Geometry: final body of the model. Coordinates: model frame, mm. A direction names the side the tool comes from. Give positions to 0.01 mm unless a question says otherwise; leave off trailing zeros. Write each loop counter-clockwise with the first axis right and the second up, starting at its lowest first coordinate (ties: lowest second). Pieces come first, ordered by that corner, then holes. Notation, with made-up numbers: (-3, -12.75) -> (43, -12.75) arc R23 cw to (43, 25.25) -> close; hole circle Ø6 at (35, 50.25). An arc over 180 degrees is marked (long way). Use CSV: the item, a comma, the result in double quotes. Start each with the question number.
1) Section D-D (z = 3.5). Output: boundary loops of the cut face in (x, y), plus the area to 3 significant figures.
2) Section A-A (z = 6). Output: boundary loops of the cut face in (x, y), plus the area to 3 significant figures.
3) Section C-C (x = 6.5). Output: boundary loops of the cut face in (y, z), plus the area to 3 significant figures.
4) Contact query for flat-ended pins moving along their axis: P1, Ø1.5, axis at x = -9, z = 10.5, coming from the -Y side; P2, Ø4, axis at x = 10, y = 6, coming from the +Z side; P3, Ø4, axis at x = -7.53, y = 0, coming from the -Z side; P4, Ø2.5, axis at y = -8, z = -3.5, coming from the +X side. Output: stop coordinate, or through.
5) Material intervals for line 1 (X direction, y = 10, z = 6.5); line 2 (X direction, y = 7.25, z = 6.75); line 3 (X direction, y = -0.75, z = 1), sorted ascending. Write a range as [from, to].
6) Draft query along X for faces 4 (the face through (9.432, -3, 1)), 5 (the face through (0.332, -7.4, -4.5)), 6 (the face through (-3.81, -10, -1)). Return one class per face: pulls with the +X half, pulls with the -X half, needs draft (parallel to the pull), parting line crosses it, or undercut.
7) Section B-B (y = 0). Output: boundary loops of the cut face in (x, z).
8) Set-up query: faces 1 (the face through (11.34, 8.13, 2.98)), 2 (the face through (3, -8.46, -1)), 3 (the face through (0, -9, -2.54)). Return all of +Z, -Z, +X, -X, +Y, -Y with unobstructed straight access to the full face (end or side cutting, diameter ignored); none if empty.
```python
from build123d import *

# Parameters (mm, degrees)
IZIM1_R                     = 1.900647948
IZIM1_R_2                   = 1.75
Y_KSEKLIK_EKSTR_ZYON1_DEPTH = 1.7
IZIM2_R                     = 2
Y_KSEKLIK_EKSTR_ZYON2_DEPTH = 2.6
IZIM3_W                     = 4.100055298
IZIM3_H                     = 6.937365011
Y_KSEKLIK_EKSTR_ZYON3_DEPTH = 8.5
IZIM4_W                     = 5.8
IZIM4_H                     = 6.937365011
Y_KSEKLIK_EKSTR_ZYON4_DEPTH = 0.6
Y_KSEKLIK_EKSTR_ZYON6_DEPTH = 2.54
IZIM6_W                     = 18.863930886
IZIM6_H                     = 1.7
Y_KSEKLIK_EKSTR_ZYON7_DEPTH = 0.01
KES_EKSTR_ZYON1_DEPTH       = 5.9
KES_EKSTR_ZYON1_DEPTH_BACK  = 0.1
IZIM7_W                     = 6.75
IZIM7_H                     = 0.75
IZIM8_W                     = 0.664910116
IZIM8_H                     = 0.664910116
IZIM11_W                    = 0.65
IZIM11_H                    = 0.6
Y_KSEKLIK_EKSTR_ZYON8_DEPTH = 1
Y_KSEKLIK_EKSTR_ZYON9_DEPTH = 1.5


with BuildPart() as part:
    # Çizim1 → Yükseklik-Ekstrüzyon1 (new body)
    with BuildSketch(Plane.XY):
        with BuildLine():
            Line((-9.431965443, -11), (9.431965443, -11))
            Line((9.431965443, -11), (9.431965443, 4.062634989))
            ThreePointArc((9.431965443, 4.062634989), (12.900647948, 7.531317495), (9.431965443, 11))
            Line((9.431965443, 11), (-9.431965443, 11))
            ThreePointArc((-9.431965443, 11), (-12.900647948, 7.531317495), (-9.431965443, 4.062634989))
            Line((-9.431965443, 4.062634989), (-9.431965443, -11))
        make_face()
        with Locations((9.431965443, 7.531317495)):
            Circle(IZIM1_R, mode=Mode.SUBTRACT)
        with Locations(Location((-9.431965443, 7.531317495, 0), (0, 0, 180))):
            Circle(IZIM1_R, mode=Mode.SUBTRACT)
        with Locations((7.531317495, 0)):
            Circle(IZIM1_R_2, mode=Mode.SUBTRACT)
        with Locations(Location((-7.531317495, 0, 0), (0, 0, 180))):
            Circle(IZIM1_R_2, mode=Mode.SUBTRACT)
    extrude(amount=Y_KSEKLIK_EKSTR_ZYON1_DEPTH)

    # Çizim2 → Yükseklik-Ekstrüzyon2 (add)
    with BuildSketch(Plane.XY.offset(1.7)):
        with BuildLine():
            Line((-9.431965443, 11), (9.431965443, 11))
            ThreePointArc((9.431965443, 11), (12.900647948, 7.531317495), (9.431965443, 4.062634989))
            Line((9.431965443, 4.062634989), (-9.431965443, 4.062634989))
            ThreePointArc((-9.431965443, 4.062634989), (-12.900647948, 7.531317495), (-9.431965443, 11))
        make_face()
        with Locations((-9.431965443, 7.531317495)):
            Circle(IZIM2_R, mode=Mode.SUBTRACT)
        with Locations((9.431965443, 7.531317495)):
            Circle(IZIM2_R, mode=Mode.SUBTRACT)
    extrude(amount=Y_KSEKLIK_EKSTR_ZYON2_DEPTH)

    # Çizim3 → Yükseklik-Ekstrüzyon3 (add)
    with BuildSketch(Plane.XY.offset(4.3)):
        with Locations((4.950027649, 7.531317494)):
            Rectangle(IZIM3_W, IZIM3_H)
        with Locations((-4.950027649, 7.531317494)):
            Rectangle(IZIM3_W, IZIM3_H)
    extrude(amount=Y_KSEKLIK_EKSTR_ZYON3_DEPTH)

    # Çizim4 → Yükseklik-Ekstrüzyon4 (add)
    with BuildSketch(Plane.XY.offset(4.3)):
        with Locations((0, 7.531317494)):
            Rectangle(IZIM4_W, IZIM4_H)
    extrude(amount=Y_KSEKLIK_EKSTR_ZYON4_DEPTH)

    # Çizim5 → Yükseklik-Ekstrüzyon6 (add)
    with BuildSketch(Plane(origin=(0, 0, 0), x_dir=(-1, 0, 0), z_dir=(0, 0, -1))):
        Polygon((-1.27, -10.75), (-1.27, -8.71), (-1.52, -8.46), (-3.56, -8.46), (-3.81, -8.71), (-3.81, -10.75), (-3.56, -11), (-1.52, -11), align=None)
        Polygon((1.27, -8.71), (1.02, -8.46), (-1.02, -8.46), (-1.27, -8.71), (-1.27, -10.75), (-1.02, -11), (1.02, -11), (1.27, -10.75), align=None)
        Polygon((1.52, -8.46), (1.27, -8.71), (1.27, -10.75), (1.52, -11), (3.56, -11), (3.81, -10.75), (3.81, -8.71), (3.56, -8.46), align=None)
    extrude(amount=Y_KSEKLIK_EKSTR_ZYON6_DEPTH)

    # Çizim6 → Yükseklik-Ekstrüzyon7 (add)
    with BuildSketch(Plane.XZ.offset(11)):
        with Locations((0, 0.85)):
            Rectangle(IZIM6_W, IZIM6_H)
    extrude(amount=Y_KSEKLIK_EKSTR_ZYON7_DEPTH)

    # Çizim7 → Kes-Ekstrüzyon1 (cut, two sides: drawn at the far end of the back side and taken through both)
    with BuildSketch(Plane.ZY.offset(-2.9).offset(-KES_EKSTR_ZYON1_DEPTH_BACK)):
        with Locations((8.275, 7.531317495)):
            Rectangle(IZIM7_W, IZIM7_H)
    extrude(amount=KES_EKSTR_ZYON1_DEPTH + KES_EKSTR_ZYON1_DEPTH_BACK, mode=Mode.SUBTRACT)

    # Süpür1: sweep along a path in Çizim9
    with BuildLine(Plane(origin=(0, 0, 0), x_dir=(0, 0, -1), z_dir=(1, 0, 0))) as s_p_r1_path:
        Line((2.54, -9.73), (4.04, -9.73))
        ThreePointArc((4.04, -9.73), (4.393553391, -9.583553391), (4.54, -9.23))
        Line((4.54, -9.23), (4.54, -3.305))
    # Çizim8 → Süpür1 (sweep)
    with BuildSketch(Plane(origin=(0, 0, -2.54), x_dir=(-1, 0, 0), z_dir=(0, 0, -1))):
        with Locations((2.54, -9.73)):
            Rectangle(IZIM8_W, IZIM8_H)
        with Locations((0, -9.73)):
            Rectangle(IZIM8_W, IZIM8_H)
        with Locations((-2.54, -9.73)):
            Rectangle(IZIM8_W, IZIM8_H)
    sweep(path=s_p_r1_path.line)

    # Çizim11 → Yükseklik-Ekstrüzyon8 (add)
    with BuildSketch(Plane.XY.offset(1.7)):
        with Locations((-2.54, -9.73)):
            Rectangle(IZIM11_W, IZIM11_H)
        with Locations((0, -9.73)):
            Rectangle(IZIM11_W, IZIM11_H)
        with Locations((2.54, -9.73)):
            Rectangle(IZIM11_W, IZIM11_H)
    extrude(amount=Y_KSEKLIK_EKSTR_ZYON8_DEPTH)

    # Çizim12 → Yükseklik-Ekstrüzyon9 (add)
    with BuildSketch(Plane(origin=(0, 0, 0), x_dir=(-1, 0, 0), z_dir=(0, 0, -1))):
        Polygon((-4.998159683, 0), (-4.998159683, 2.331223734), (-1.20341454, 2.331223734), (-1.20341454, -3.045965908), (-4.998159683, -3.045965908), align=None)
    extrude(amount=Y_KSEKLIK_EKSTR_ZYON9_DEPTH)


solid = part.part
```
Answers follow:
1,outline,"(-9.43, 4.06) -> (9.43, 4.06) arc R3.47 ccw to (9.43, 11) -> (-9.43, 11) arc R3.47 ccw to start; hole circle Ø4 at (-9.43, 7.53); hole circle Ø4 at (9.43, 7.53)"
1,area,"144 mm^2"
2,outline,"(-7, 4.06) -> (-2.9, 4.06) -> (-2.9, 7.16) -> (-3, 7.16) -> (-3, 7.91) -> (-2.9, 7.91) -> (-2.9, 11) -> (-7, 11) -> close; (2.9, 4.06) -> (7, 4.06) -> (7, 11) -> (2.9, 11) -> (2.9, 7.91) -> (3, 7.91) -> (3, 7.16) -> (2.9, 7.16) -> close"
2,area,"56.7 mm^2"
3,outline,"(-11.01, 0) -> (-1.41, 0) -> (-1.41, 1.7) -> (-11.01, 1.7) -> close; (1.41, 0) -> (11, 0) -> (11, 12.8) -> (4.06, 12.8) -> (4.06, 1.7) -> (1.41, 1.7) -> close"
3,area,"110 mm^2"
4,P1,"passes through"
4,P2,"stops at z = 4.3"
4,P3,"stops at z = 0"
4,P4,"stops at x = 3.81"
5,line 1,"x = [-7, -2.9], [2.9, 7]"
5,line 2,"x = [-7, -3], [3, 7]"
5,line 3,"x = [-9.43, -9.11], [-5.95, 5.95], [9.11, 9.43]"
6,face 4,"pulls with the +X half"
6,face 5,"undercut"
6,face 6,"pulls with the -X half"
7,outline,"(-9.43, 0) -> (-9.28, 0) -> (-9.28, 1.7) -> (-9.43, 1.7) -> close; (-5.78, 0) -> (1.2, 0) -> (1.2, -1.5) -> (5, -1.5) -> (5, 0) -> (5.78, 0) -> (5.78, 1.7) -> (-5.78, 1.7) -> close; (9.28, 0) -> (9.43, 0) -> (9.43, 1.7) -> (9.28, 1.7) -> close"
8,face 1,"+Z"
8,face 2,"+X, -X"
8,face 3,"none"
